For this review, take the finished solid that the model builds, in its own axes (mm). Face numbers are marked on the shaded views. A direction names the side the tool comes from. Round coordinates to 2 decimals unless told otherwise and drop trailing zeros. Order: outer loops, then holes, each group sorted by start corner. A loop starts at its lowest first (then second) coordinate and runs counter-clockwise, first axis right, second up. Notation, with made-up numbers: M -5,19 L 34,19 A24 cw 34,40 Z; hole C 51,67.25 d7. An arc over 180 degrees is marked long. Answer as a JSON object with one key per item and string values.
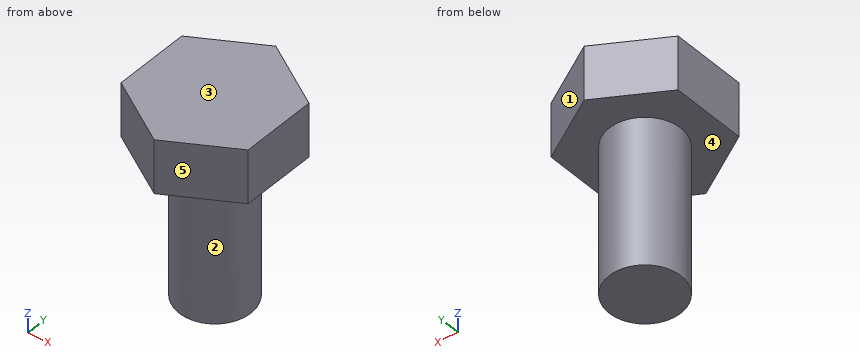
from build123d import *

# Parameters (mm, degrees)
EXTRUDE_1_DEPTH = 2.9
SKETCH_4_R      = 1.925
EXTRUDE_2_DEPTH = 7.95


with BuildPart() as part:
    # Эскиз1 → Бобышка-Вытянуть1 (new body)
    with BuildSketch(Plane.XY):
        Polygon((3.380947783, -1.962353809), (3.456334009, 1.991776974), (0.069649414, 4.034128753), (-3.392421407, 2.122349748), (-3.467807633, -1.831781035), (-0.081123038, -3.874132814), align=None)
    extrude(amount=-EXTRUDE_1_DEPTH)

    # Эскиз4 → Бобышка-Вытянуть2 (add)
    with BuildSketch(Plane(origin=(0, 0, -2.9), x_dir=(-1, 0, 0), z_dir=(0, 0, -1))):
        with Locations((0.005736812, 0.07999797)):
            Circle(SKETCH_4_R)
    extrude(amount=EXTRUDE_2_DEPTH)


solid = part.part
1) Add section A-A on z = -2.25. State the section outline as (x, y) points, and give its area (3 significant figures).
Geometry check:
{"outline": "M -3.47,-1.83 L -0.08,-3.87 L 3.38,-1.96 L 3.46,1.99 L 0.07,4.03 L -3.39,2.12 Z", "area": "40.6 mm²"}
2) Add section C-C on y = 0.25. State the section outline as (x, z) points.
Geometry check:
{"outline": "M -3.43,-2.9 L -1.92,-2.9 L -1.92,-10.85 L 1.91,-10.85 L 1.91,-2.9 L 3.42,-2.9 L 3.42,0 L -3.43,0 Z"}
3) Add section D-D on z = -9.75. State the section outline as (x, y) points (3 decimals).
Geometry check:
{"outline": "C -0.006,0.08 d3.85"}
4) Insertion check: P1, Ø1.5, axis at x = 2, z = -9.5, coming from the -Y side; P2, Ø4, axis at x = 1.5, z = -6.5, coming from the -Y side (3 decimals); P3, Ø3, axis at y = 2.5, z = -8.5, coming from the +X side. Each pin has a flat end and moves straight along its axis. Give the tip position at first contact, or say it passes through.
Geometry check:
{"P1": "stops at y = -1.38", "P2": "stops at y = -1.845", "P3": "stops at x = 1.69"}
5) Machinability: for the marked faces 1 and 2, which of the approach directions +Z, -Z, +X, -X, +Y, -Y give a long, thin tool a straight path to every point of the face, cutting with its end or side? Answer none if there is none.
Geometry check:
{"face 1": "+Z, -Z, +X, +Y", "face 2": "-Z"}
6) For L1, parallel to Z at x = 0, y = -3.25; L2, parallel to Y at x = 0.25, z = -4; L3, parallel to X at y = 0.25, z = -1.25, list the stretches that pass through material, from the lowest coordinate up.
Geometry check:
{"L1": "z = -2.9 to 0", "L2": "y = -1.83 to 1.99", "L3": "x = -3.43 to 3.42"}
7) Mouldability with a two-part tool opening along Z and no side actions: class the marked faces 3, 4 and 5 as +Z half, -Z half, draft (parallel to the pull), parting line (faces both ways), or undercut.
Geometry check:
{"face 3": "+Z half", "face 4": "-Z half", "face 5": "draft"}
8) Add section B-B on x = 0.75. State the section outline as (y, z) points.
Geometry check:
{"outline": "M -3.42,-2.9 L -1.69,-2.9 L -1.69,-10.85 L 1.85,-10.85 L 1.85,-2.9 L 3.62,-2.9 L 3.62,0 L -3.42,0 Z"}
